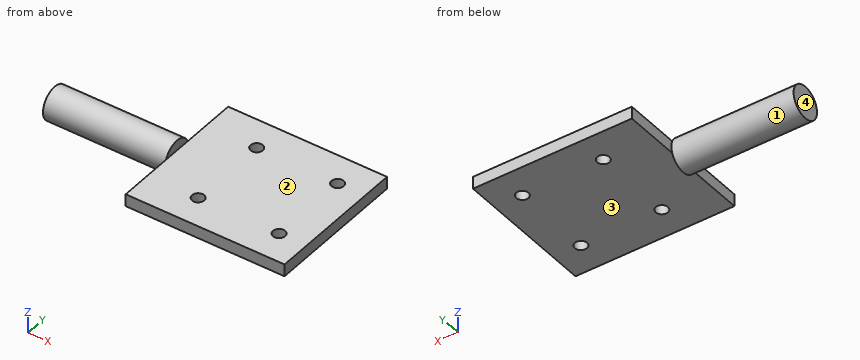
from build123d import *

# Parameters (mm, degrees)
SKETCH_1_W           = 34
SKETCH_1_H           = 35
EXTRUDE_1_DEPTH      = 3
SKETCH_2_W           = 5
SKETCH_2_H           = 5
EXTRUDE_2_DEPTH      = 3
SKETCH_7_R           = 1.5
CUT_EXTRUDE_7_DEPTH  = 3
SKETCH_14_R          = 4
EXTRUDE_6_DEPTH      = 25
EXTRUDE_START        = 5
SKETCH_16_R          = 4
EXTRUDE_7_DEPTH      = 5
CUT_EXTRUDE_START    = -5
CUT_EXTRUDE_9_DEPTH  = 5
EXTRUDE_8_DEPTH      = 5
SKETCH_19_W          = 5
SKETCH_19_H          = 2.5
CUT_EXTRUDE_10_DEPTH = 59.857879676
SKETCH_20_R          = 4
EXTRUDE_9_DEPTH      = 29.5
SKETCH_21_W          = 26.980293682
SKETCH_21_H          = 10.390157326
CUT_EXTRUDE_11_DEPTH = 85.305990297


with BuildPart() as part:
    # 草图1 → 凸台-拉伸1 (new body)
    with BuildSketch(Plane.XY):
        Rectangle(SKETCH_1_W, SKETCH_1_H)
    extrude(amount=EXTRUDE_1_DEPTH)

    # 草图2 → 凸台-拉伸2 (add)
    with BuildSketch(Plane.XY.offset(3)):
        with Locations((-19.5, 2.5)):
            Rectangle(SKETCH_2_W, SKETCH_2_H)
        with Locations((-19.5, -2.5)):
            Rectangle(SKETCH_2_W, SKETCH_2_H)
    extrude(amount=-EXTRUDE_2_DEPTH)

    # 草图7 → 切除-拉伸7 (cut)
    with BuildSketch(Plane.XY.offset(3)):
        with Locations((10.27515824, 10)):
            Circle(SKETCH_7_R)
        with Locations((10.27515824, -10)):
            Circle(SKETCH_7_R)
        with Locations((-9.593631375, 10)):
            Circle(SKETCH_7_R)
        with Locations((-9.593631375, -10)):
            Circle(SKETCH_7_R)
    extrude(amount=-CUT_EXTRUDE_7_DEPTH, mode=Mode.SUBTRACT)

    # 草图14 → 凸台-拉伸6 (add)
    with BuildSketch(Plane.ZY.offset(22)):
        with Locations(Location((1.5, 0, 0), (0, 0, 112.024312837))):
            Circle(SKETCH_14_R)
    extrude(amount=EXTRUDE_6_DEPTH)

    # 草图16 → 凸台-拉伸7 (add)
    with BuildSketch(Plane(origin=(-22, 0, 0), x_dir=(0, 0, -1), z_dir=(1, 0, 0)).offset(EXTRUDE_START)):
        with Locations(Location((-1.5, 0, 0), (0, 0, 67.975687163))):
            Circle(SKETCH_16_R)
    extrude(amount=-EXTRUDE_7_DEPTH)

    # 草图17 → 切除-拉伸9 (cut)
    with BuildSketch(Plane.ZY.offset(22).offset(CUT_EXTRUDE_START)):
        with BuildLine():
            Line((3, 3.708099244), (3, 5))
            Line((3, 5), (0, 5))
            Line((0, 5), (0, 3.708099244))
            ThreePointArc((0, 3.708099244), (1.5, 4), (3, 3.708099244))
        make_face()
        with BuildLine():
            Line((0, -3.708099244), (0, -5))
            Line((0, -5), (3, -5))
            Line((3, -5), (3, -3.708099244))
            ThreePointArc((3, -3.708099244), (1.5, -4), (0, -3.708099244))
        make_face()
    extrude(amount=CUT_EXTRUDE_9_DEPTH, mode=Mode.SUBTRACT)

    # 草图18 → 凸台-拉伸8 (add)
    with BuildSketch(Plane.ZY.offset(17)):
        with BuildLine():
            Line((3, -17.5), (3, -3.708099244))
            ThreePointArc((3, -3.708099244), (1.5, -4), (0, -3.708099244))
            Line((0, -3.708099244), (0, -17.5))
            Line((0, -17.5), (3, -17.5))
        make_face()
        with BuildLine():
            Line((0, 17.5), (0, 3.708099244))
            ThreePointArc((0, 3.708099244), (1.5, 4), (3, 3.708099244))
            Line((3, 3.708099244), (3, 17.5))
            Line((3, 17.5), (0, 17.5))
        make_face()
    extrude(amount=EXTRUDE_8_DEPTH)

    # 草图19 → 切除-拉伸10 (cut, through all)
    with BuildSketch(Plane.XZ.offset(17.5)):
        with Locations((-19.5, 4.25)):
            Rectangle(SKETCH_19_W, SKETCH_19_H)
        with Locations((-19.5, -1.25)):
            Rectangle(SKETCH_19_W, SKETCH_19_H)
    extrude(amount=-CUT_EXTRUDE_10_DEPTH, mode=Mode.SUBTRACT)

    # 草图20 → 凸台-拉伸9 (add)
    with BuildSketch(Plane.ZY.offset(47)):
        with Locations(Location((1.5, 0, 0), (0, 0, 112.024312837))):
            Circle(SKETCH_20_R)
    extrude(amount=EXTRUDE_9_DEPTH)

    # 草图21 → 切除-拉伸11 (cut, through all)
    with BuildSketch(Plane.XZ.offset(17.5)):
        with Locations((-65.490146841, 2.695078663)):
            Rectangle(SKETCH_21_W, SKETCH_21_H)
    extrude(amount=-CUT_EXTRUDE_11_DEPTH, mode=Mode.SUBTRACT)


solid = part.part
Geometry check sheet. Reference: the model listing, model coordinates, mm. Face numbers are marked on the shaded views. A direction names the side the tool comes from. Give positions to 0.01 mm unless a question says otherwise; leave off trailing zeros. Write each loop counter-clockwise with the first axis right and the second up, starting at its lowest first coordinate (ties: lowest second). Pieces come first, ordered by that corner, then holes. Notation, with made-up numbers: (78.5, 35) - (90.5, 35) arc R25 cw to (90.5, 53) - close; hole circle Ø4 at (6, -35.5). An arc over 180 degrees is marked (long way). Put each result on its own line as item: value.
1. Sectioned sample at B-B, the plane z = 1.5. Enter the section's corners in (x, y), plus the area to 3 significant figures.
Ans:
outline: (-52, -4) - (-22, -4) - (-22, -17.5) - (17, -17.5) - (17, 17.5) - (-22, 17.5) - (-22, 4) - (-52, 4) - close; hole circle Ø3 at (-9.59, -10); hole circle Ø3 at (-9.59, 10); hole circle Ø3 at (10.28, -10); hole circle Ø3 at (10.28, 10)
area: 1,580 mm²
2. Sectioned sample at D-D, the plane y = 0. Enter the section's corners in (x, z), plus the area to 3 significant figures.
Ans:
outline: (-52, -2.5) - (-22, -2.5) - (-22, 0) - (17, 0) - (17, 3) - (-22, 3) - (-22, 5.5) - (-52, 5.5) - close
area: 357 mm²
3. Sectioned sample at C-C, the plane x = -10. Enter the section's corners in (y, z).
Ans:
outline: (-17.5, 0) - (-11.44, 0) - (-11.44, 3) - (-17.5, 3) - close; (-8.56, 0) - (8.56, 0) - (8.56, 3) - (-8.56, 3) - close; (11.44, 0) - (17.5, 0) - (17.5, 3) - (11.44, 3) - close
4. Set-up check for the marked faces 1, 2, 3 and 4: record each of +Z, -Z, +X, -X, +Y, -Y from which the full face is reachable in a straight line by a thin tool's end or side.
Ans:
face 1: -X
face 2: +Z, +X, +Y, -Y
face 3: -Z, +X, +Y, -Y
face 4: +Z, -Z, -X, +Y, -Y
5. Sectioned sample at A-A, the plane y = -10. Enter the section's corners in (x, z), plus the area to 3 significant figures.
Ans:
outline: (-22, 0) - (-11.09, 0) - (-11.09, 3) - (-22, 3) - close; (-8.09, 0) - (8.78, 0) - (8.78, 3) - (-8.09, 3) - close; (11.78, 0) - (17, 0) - (17, 3) - (11.78, 3) - close
area: 99.0 mm²
6. Thickness scan on line 1 (X direction, y = -9.5, z = 0.25); line 2 (X direction, y = -15.5, z = 2.75); line 3 (Z direction, x = 8, y = 10). Record the ranges inside material, lowest first.
Ans:
line 1: x = -22 to -11.01, -8.18 to 8.86, 11.69 to 17
line 2: x = -22 to 17
line 3: z = 0 to 3
7. Go/stop test with flat-tipped pins: pin 1 (4 mm diameter, centred on x = -32, z = 1.5, fed in from -Y); pin 2 (17.5 mm diameter, centred on x = 6, y = -7, fed in from +Z); pin 3 (3 mm diameter, centred on x = -42.5, y = -0.5, fed in from +Z); pin 4 (2.5 mm diameter, centred on x = 10.28, y = 10, fed in from -Z). Record where each tip stops, or that it passes through.
Ans:
pin 1: stops at y = -4
pin 2: stops at z = 3
pin 3: stops at z = 5.5
pin 4: passes through
